For this review, take the finished solid that the model builds, in its own axes (mm). A direction names the side the tool comes from. Give positions to 0.01 mm unless a question says otherwise; leave off trailing zeros. Order: outer loops, then holes, each group sorted by start corner. A loop starts at its lowest first (then second) coordinate and runs counter-clockwise, first axis right, second up. Notation, with made-up numbers: (75.5, -39.75) - (110.5, -39.75) arc R20 ccw to (110.5, -17.75) - close; hole circle Ø10 at (87, -7). An arc over 180 degrees is marked (long way). One line per item, written item: value.
```python
from build123d import *

# Parameters (mm, degrees)
F0_R     = 4
F1_DEPTH = 5
F3_DEPTH = 10


with BuildPart() as f1:
    # F0 (on Front) → F1 (new body, symmetric)
    with BuildSketch(Plane.XZ):
        with BuildLine():
            Line((-12.679406, 22.584124), (-10.90092, 18.589579))
            ThreePointArc((-10.90092, 18.589579), (-12.666772, 17.434316), (-14.311171, 16.111887))
            Line((-14.311171, 16.111887), (-17.560627, 19.03771))
            ThreePointArc((-17.560627, 19.03771), (-21.030999, 18.936396), (-20.769004, 15.474445))
            Line((-20.769004, 15.474445), (-17.519549, 12.548622))
            ThreePointArc((-17.519549, 12.548622), (-18.662847, 10.775), (-19.6272, 8.898063))
            Line((-19.6272, 8.898063), (-23.785765, 10.249263))
            ThreePointArc((-23.785765, 10.249263), (-26.914899, 8.745181), (-25.267454, 5.689094))
            Line((-25.267454, 5.689094), (-21.108888, 4.337894))
            ThreePointArc((-21.108888, 4.337894), (-21.431947, 2.252588), (-21.549508, 0.145684))
            Line((-21.549508, 0.145684), (-25.898128, -0.311375))
            ThreePointArc((-25.898128, -0.311375), (-28.14497, -2.958156), (-25.39693, -5.079953))
            Line((-25.39693, -5.079953), (-21.04831, -4.622895))
            ThreePointArc((-21.04831, -4.622895), (-20.495268, -6.659316), (-19.74571, -8.631886))
            Line((-19.74571, -8.631886), (-23.53247, -10.818173))
            ThreePointArc((-23.53247, -10.818173), (-24.508519, -14.15), (-21.135047, -14.97063))
            Line((-21.135047, -14.97063), (-17.348287, -12.784343))
            ThreePointArc((-17.348287, -12.784343), (-16.014771, -14.419765), (-14.527699, -15.916924))
            Line((-14.527699, -15.916924), (-17.097834, -19.45441))
            ThreePointArc((-17.097834, -19.45441), (-16.634323, -22.895181), (-13.218722, -22.27275))
            Line((-13.218722, -22.27275), (-10.648588, -18.735263))
            ThreePointArc((-10.648588, -18.735263), (-8.765175, -19.686905), (-6.797718, -20.449781))
            Line((-6.797718, -20.449781), (-7.706827, -24.726804))
            ThreePointArc((-7.706827, -24.726804), (-5.883901, -27.681577), (-3.01676, -25.723708))
            Line((-3.01676, -25.723708), (-2.107651, -21.446685))
            ThreePointArc((-2.107651, -21.446685), (0, -21.55), (2.107651, -21.446685))
            Line((2.107651, -21.446685), (3.01676, -25.723708))
            ThreePointArc((3.01676, -25.723708), (5.883901, -27.681577), (7.706827, -24.726804))
            Line((7.706827, -24.726804), (6.797718, -20.449781))
            ThreePointArc((6.797718, -20.449781), (8.765175, -19.686905), (10.648588, -18.735263))
            Line((10.648588, -18.735263), (13.218722, -22.27275))
            ThreePointArc((13.218722, -22.27275), (16.634323, -22.895181), (17.097834, -19.45441))
            Line((17.097834, -19.45441), (14.527699, -15.916924))
            ThreePointArc((14.527699, -15.916924), (16.014771, -14.419765), (17.348287, -12.784343))
            Line((17.348287, -12.784343), (21.135047, -14.97063))
            ThreePointArc((21.135047, -14.97063), (24.508519, -14.15), (23.53247, -10.818173))
            Line((23.53247, -10.818173), (19.74571, -8.631886))
            ThreePointArc((19.74571, -8.631886), (20.495268, -6.659316), (21.04831, -4.622895))
            Line((21.04831, -4.622895), (25.39693, -5.079953))
            ThreePointArc((25.39693, -5.079953), (28.14497, -2.958156), (25.898128, -0.311375))
            Line((25.898128, -0.311375), (21.549508, 0.145684))
            ThreePointArc((21.549508, 0.145684), (21.431947, 2.252588), (21.108888, 4.337894))
            Line((21.108888, 4.337894), (25.267454, 5.689094))
            ThreePointArc((25.267454, 5.689094), (26.914899, 8.745181), (23.785765, 10.249263))
            Line((23.785765, 10.249263), (19.6272, 8.898063))
            ThreePointArc((19.6272, 8.898063), (18.662847, 10.775), (17.519549, 12.548622))
            Line((17.519549, 12.548622), (20.769004, 15.474445))
            ThreePointArc((20.769004, 15.474445), (21.030999, 18.936396), (17.560627, 19.03771))
            Line((17.560627, 19.03771), (14.311171, 16.111887))
            ThreePointArc((14.311171, 16.111887), (12.666772, 17.434316), (10.90092, 18.589579))
            Line((10.90092, 18.589579), (12.679406, 22.584124))
            ThreePointArc((12.679406, 22.584124), (11.510647, 25.853336), (8.299097, 24.534364))
            Line((8.299097, 24.534364), (6.520611, 20.539818))
            ThreePointArc((6.520611, 20.539818), (4.480497, 21.079081), (2.397423, 21.416229))
            Line((2.397423, 21.416229), (2.397423, 25.788803))
            ThreePointArc((2.397423, 25.788803), (0, 28.3), (-2.397423, 25.788803))
            Line((-2.397423, 25.788803), (-2.397423, 21.416229))
            ThreePointArc((-2.397423, 21.416229), (-4.480497, 21.079081), (-6.520611, 20.539818))
            Line((-6.520611, 20.539818), (-8.299097, 24.534364))
            ThreePointArc((-8.299097, 24.534364), (-11.510647, 25.853336), (-12.679406, 22.584124))
        make_face()
        Circle(F0_R, mode=Mode.SUBTRACT)
    extrude(amount=F1_DEPTH, both=True)

    # F2 (on face) → F3 (cut)
    with BuildSketch(Plane.XZ.offset(5)):
        with BuildLine():
            ThreePointArc((-5.755287, 18.159823), (-13.470384, 13.470384), (-18.159823, 5.755287))
            ThreePointArc((-18.159823, 5.755287), (-18.247266, 5.382134), (-18.276644, 5))
            Line((-18.276644, 5), (-4.153312, 5))
            ThreePointArc((-4.153312, 5), (-3.887479, 5.209367), (-3.611111, 5.404616))
            ThreePointArc((-3.611111, 5.404616), (-2.795207, 6.304803), (-2.5, 7.483315))
            Line((-2.5, 7.483315), (-2.5, 15.776644))
            ThreePointArc((-2.5, 15.776644), (-3.523216, 17.793847), (-5.755287, 18.159823))
        make_face()
        with BuildLine():
            Line((-4.153312, 5), (-18.276644, 5))
            ThreePointArc((-18.276644, 5), (-17.544411, 3.232233), (-15.776644, 2.5))
            Line((-15.776644, 2.5), (-7.483315, 2.5))
            ThreePointArc((-7.483315, 2.5), (-6.304803, 2.795207), (-5.404616, 3.611111))
            ThreePointArc((-5.404616, 3.611111), (-4.829156, 4.350776), (-4.153312, 5))
        make_face()
        with BuildLine():
            ThreePointArc((5.755287, 18.159823), (3.523216, 17.793847), (2.5, 15.776644))
            Line((2.5, 15.776644), (2.5, 7.483315))
            ThreePointArc((2.5, 7.483315), (2.795207, 6.304803), (3.611111, 5.404616))
            ThreePointArc((3.611111, 5.404616), (4.596194, 4.596194), (5.404616, 3.611111))
            ThreePointArc((5.404616, 3.611111), (6.304803, 2.795207), (7.483315, 2.5))
            Line((7.483315, 2.5), (15.776644, 2.5))
            ThreePointArc((15.776644, 2.5), (17.793847, 3.523216), (18.159823, 5.755287))
            ThreePointArc((18.159823, 5.755287), (13.470384, 13.470384), (5.755287, 18.159823))
        make_face()
        with BuildLine():
            Line((-7.483315, -2.5), (-15.776644, -2.5))
            ThreePointArc((-15.776644, -2.5), (-17.793847, -3.523216), (-18.159823, -5.755287))
            ThreePointArc((-18.159823, -5.755287), (-13.470384, -13.470384), (-5.755287, -18.159823))
            ThreePointArc((-5.755287, -18.159823), (-3.523216, -17.793847), (-2.5, -15.776644))
            Line((-2.5, -15.776644), (-2.5, -7.483315))
            ThreePointArc((-2.5, -7.483315), (-2.795207, -6.304803), (-3.611111, -5.404616))
            ThreePointArc((-3.611111, -5.404616), (-4.596194, -4.596194), (-5.404616, -3.611111))
            ThreePointArc((-5.404616, -3.611111), (-6.304803, -2.795207), (-7.483315, -2.5))
        make_face()
        with BuildLine():
            ThreePointArc((5.404616, -3.611111), (4.596194, -4.596194), (3.611111, -5.404616))
            ThreePointArc((3.611111, -5.404616), (2.795207, -6.304803), (2.5, -7.483315))
            Line((2.5, -7.483315), (2.5, -15.776644))
            ThreePointArc((2.5, -15.776644), (3.523216, -17.793847), (5.755287, -18.159823))
            ThreePointArc((5.755287, -18.159823), (13.470384, -13.470384), (18.159823, -5.755287))
            ThreePointArc((18.159823, -5.755287), (17.793847, -3.523216), (15.776644, -2.5))
            Line((15.776644, -2.5), (7.483315, -2.5))
            ThreePointArc((7.483315, -2.5), (6.304803, -2.795207), (5.404616, -3.611111))
        make_face()
    extrude(amount=-F3_DEPTH, mode=Mode.SUBTRACT)


solid = f1.part
```
(1) Draft analysis for pull direction Z (two halves, no side actions). For faces 1 (the face through (-2.397, 0, 24)), 2 (the face through (7.422, -0.07, 22.565)), 3 (the face through (15.83, -0.07, -17.71)), 4 (the face through (-20.504, -0.07, -6.631)), state which applies: pulls with the +Z half, pulls with the -Z half, needs draft (parallel to the pull), parting line crosses it, or undercut.
Answers below:
face 1: needs draft
face 2: pulls with the +Z half
face 3: undercut
face 4: undercut
(2) Machinability: for faces 5 (the face through (-19.167, -0.07, 14.032)), 6 (the face through (2.397, 0, 24)), 7 (the face through (12.691, -0.07, 17.417)), 8 (the face through (23.754, -0.07, -0.086)), which of the approach directions +Z, -Z, +X, -X, +Y, -Y give a long, thin tool a straight path to every point of the face, cutting with its end or side? Answer none if there is none.
Answers below:
face 5: -X, +Y, -Y
face 6: +Z, +Y, -Y
face 7: +Y, -Y
face 8: +X, +Y, -Y
(3) Take a section at C-C (z = 14). Write out the cut boundary in (x, y).
Answers below:
outline: (-19.13, -5) - (-12.92, -5) - (-12.92, 5) - (-19.13, 5) - close; (-2.5, -5) - (2.5, -5) - (2.5, 5) - (-2.5, 5) - close; (12.92, -5) - (19.13, -5) - (19.13, 5) - (12.92, 5) - close
(4) Take a section at B-B (z = -24). Write out the cut boundary in (x, y).
Answers below:
outline: (-7.55, -5) - (-2.65, -5) - (-2.65, 5) - (-7.55, 5) - close; (2.65, -5) - (7.55, -5) - (7.55, 5) - (2.65, 5) - close
(5) Take a section at D-D (y = 4). Give the number of separate pieces and of enclosed holes in the cut face, then the cut area to 3 significant figures.
Answers below:
separate pieces: 1
enclosed holes: 5
area: 1,130 mm^2
(6) For P1, Ø4, axis at x = -10, y = -1.5, coming from the -Z side; P2, Ø3, axis at y = 4, z = -4, coming from the +X side; P3, Ø2, axis at y = -4, z = 20, coming from the +X side; P4, Ø1.3, axis at y = -1, z = 23, coming from the -X side, all flat-tipped, find the tip position at first contact; note any pin that passes through.
Answers below:
P1: stops at z = -20.6
P2: stops at x = 28.16
P3: stops at x = 20.97
P4: stops at x = -12.93
(7) Take a section at A-A (x = 0). Write out the cut boundary in (y, z).
Answers below:
outline: (-5, -21.55) - (5, -21.55) - (5, -4) - (-5, -4) - close; (-5, 4) - (5, 4) - (5, 28.3) - (-5, 28.3) - close
(8) Wall thickness on line 1 (Z direction, x = -3.5, y = 0.5); line 2 (X direction, y = -3.25, z = 3.5); line 3 (Z direction, x = 9, y = 0.5): over which ranges is each line inside the solid? List them lowest first. Write a range as from..to.
Answers below:
line 1: z = -26.82..-17.78, -5.48..-1.94, 1.94..5.48, 17.78..21.26
line 2: x = -21.26..-17.78, -5.48..-1.94, 1.94..5.48, 17.78..21.26
line 3: z = -19.58..-16.79, -2.5..2.5, 16.79..25.51
